Geometry check sheet. Reference: the model listing, model coordinates, mm. A direction names the side the tool comes from. Round coordinates to 2 decimals unless told otherwise and drop trailing zeros. Write each loop counter-clockwise with the first axis right and the second up, starting at its lowest first coordinate (ties: lowest second). Pieces come first, ordered by that corner, then holes. Notation, with made-up numbers: M 73,61.25 L 87,61.25 A21 ccw 87,87.25 Z; hole C 64.25,36.25 d2. An arc over 180 degrees is marked long. Answer as CSV lines item,"result". Start each with the question number.
```python
from build123d import *

# Parameters (mm, degrees)
SKETCH1_R           = 4.5
BOSS_EXTRUDE1_DEPTH = 25
SKETCH2_R           = 3
BOSS_EXTRUDE2_DEPTH = 4
BOSS_EXTRUDE3_DEPTH = 1
SKETCH4_R           = 6.35
BOSS_EXTRUDE4_DEPTH = 19.54
CUT_EXTRUDE1_DEPTH  = 19.54
SKETCH7_R           = 1.5
BOSS_EXTRUDE5_DEPTH = 18


with BuildPart() as part:
    # Sketch1 → Boss-Extrude1 (new body)
    with BuildSketch(Plane(origin=(0, 0, 0), x_dir=(1, 0, 0), z_dir=(0, 1, 0))):
        Circle(SKETCH1_R)
    extrude(amount=BOSS_EXTRUDE1_DEPTH)

    # Sketch2 → Boss-Extrude2 (add)
    with BuildSketch(Plane.XZ):
        Circle(SKETCH2_R)
    extrude(amount=BOSS_EXTRUDE2_DEPTH)

    # Sketch3 → Boss-Extrude3 (add)
    with BuildSketch(Plane.XZ.offset(4)):
        with BuildLine():
            Line((0, 3), (0, 5))
            ThreePointArc((0, 5), (-3.535533906, -3.535533906), (5, 0))
            Line((5, 0), (3, 0))
            ThreePointArc((3, 0), (-2.121320344, -2.121320344), (0, 3))
        make_face()
    extrude(amount=-BOSS_EXTRUDE3_DEPTH)

    # Sketch4 → Boss-Extrude4 (add)
    with BuildSketch(Plane.XZ.offset(4)):
        Circle(SKETCH4_R)
    extrude(amount=BOSS_EXTRUDE4_DEPTH)

    # Sketch6 → Cut-Extrude1 (cut)
    with BuildSketch(Plane(origin=(6.35, 0, 0), x_dir=(0, 0, -1), z_dir=(1, 0, 0))):
        Polygon((-8.967576024, -4), (-4.76, -4), (-4.76, -14), (4.76, -23.54), (4.76, -4), (8.459767383, -4), (8.459767383, -27.476657102), (-8.967576024, -27.476657102), align=None)
    extrude(amount=-CUT_EXTRUDE1_DEPTH, mode=Mode.SUBTRACT)

    # Sketch7 → Boss-Extrude5 (add)
    with BuildSketch(Plane(origin=(0, 25, 0), x_dir=(1, 0, 0), z_dir=(0, 1, 0))):
        Circle(SKETCH7_R)
    extrude(amount=BOSS_EXTRUDE5_DEPTH)


solid = part.part
```
1) Go/stop test with flat-tipped pins: pin 1 (3 mm diameter, centred on x = 4, z = -0.5, fed in from +Y); pin 2 (5 mm diameter, centred on x = -1.5, y = -10.5, fed in from +Z); pin 3 (5 mm diameter, centred on x = 3.5, y = 18.5, fed in from -Z). Record where each tip stops, or that it passes through.
2) Access from +Z, -Z, +X, -X, +Y, -Y to the whole of each face (thin tool, end or side, straight path). Record for faces 1 (the flat face through (0, -14, -4.76)), 2 (the flat face through (-5.2, -4, 0)), 3 (the flat face through (0, 25, 2)), 4 (the flat face through (-2.3, -3, -2.2)).
3) Section check D-D, the plane y = -8.5. Record the cut outline in (x, z).
4) Section check C-C, the plane y = 8. Record the cut outline in (x, z), plus the area to 3 significant figures.
5) Section check A-A, the plane z = -3.75. Record the cut outline in (x, y), plus the area to 3 significant figures.
6) Section check B-B, the plane x = -2.25. Record the cut outline in (y, z).
7) Scan lines: line 1 (Z direction, x = 0.75, y = -4.5); line 2 (Y direction, x = 1.5, z = -3); line 3 (X direction, y = 35, z = 0). Record each from-to range of solid material in increasing order. Write a range as from..to.
Results:
1,pin 1,"stops at y = 25"
1,pin 2,"stops at z = 4.76"
1,pin 3,"stops at z = -4.39"
2,face 1,"-Z, +X, -X, -Y"
2,face 2,"-X, +Y"
2,face 3,"+Y"
2,face 4,"none"
3,outline,"M -4.2,-4.76 L 4.2,-4.76 A6.35 ccw 4.2,4.76 L -4.2,4.76 A6.35 ccw Z"
4,outline,"C 0,0 d9"
4,area,"63.6 mm^2"
5,outline,"M -5.12,-22.53 L 5.12,-22.53 L 5.12,-4 L 3.31,-4 L 3.31,-3 L -3.31,-3 L -3.31,-4 L -5.12,-4 Z; M -2.49,0 L 2.49,0 L 2.49,25 L -2.49,25 Z"
5,area,"321 mm^2"
6,outline,"M -23.54,-4.76 L -4,-4.76 L -4,-4.47 L -3,-4.47 L -3,-1.98 L 0,-1.98 L 0,-3.9 L 25,-3.9 L 25,3.9 L 0,3.9 L 0,1.98 L -3,1.98 L -3,4.47 L -4,4.47 L -4,4.76 L -14,4.76 Z"
7,line 1,"z = -4.76..4.76"
7,line 2,"y = -21.78..-3, 0..25"
7,line 3,"x = -1.5..1.5"
